from build123d import *

# Parameters (mm, degrees)
F1_DEPTH = 20.6
F2_R     = 5


with BuildPart() as f1:
    # F0 (on Front) → F1 (new body, symmetric)
    with BuildSketch(Plane.XZ):
        Polygon((-82.7489259505, 37), (-107.7489259505, 37), (-107.7489259505, -54.4), (-83.9489259505, -54.4), (-67.4489259505, -25), (-7.4489259505, -25), (-7.4489259505, 67), (-34.7489259505, 67), (-34.7489259505, 0), (-82.7489259505, 0), align=None)
    extrude(amount=F1_DEPTH, both=True)

    # F2
    f2_edges = [f1.edges().sort_by_distance(p)[0] for p in [
        (-107.748926, 0, 37),
        (-82.748926, 0, 37),
        (-95.248926, -20.6, 37),
        (-95.248926, 20.6, 37),
        (-82.748926, -20.6, 18.5),
        (-82.748926, 0, 0),
        (-82.748926, 20.6, 18.5),
        (-58.748926, 20.6, 0),
        (-58.748926, -20.6, 0),
        (-34.748926, 0, 0),
        (-34.748926, 0, 67),
        (-21.098926, -20.6, 67),
        (-21.098926, 20.6, 67),
        (-7.448926, 0, 67),
        (-34.748926, -20.6, 33.5),
        (-7.448926, -20.6, 21),
        (-7.448926, 20.6, 21),
        (-107.748926, -20.6, -8.7),
        (-107.748926, 20.6, -8.7),
        (-34.748926, 20.6, 33.5),
    ]]
    fillet(f2_edges, radius=F2_R)


solid = f1.part
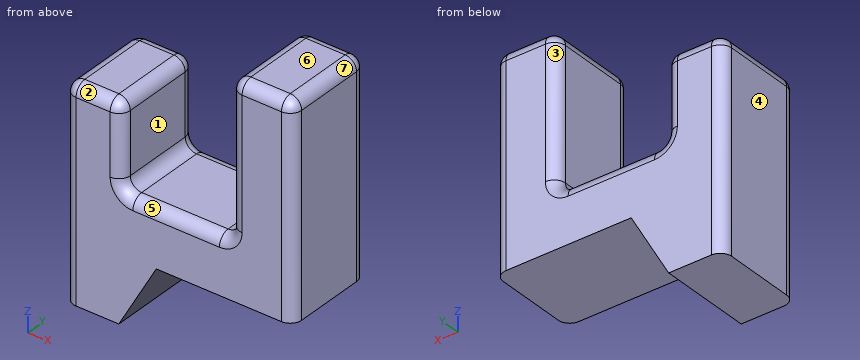
Can you work these out from the model? Positions are in its coordinate system, mm. Face numbers are marked on the shaded views. A direction names the side the tool comes from. Give positions to 0.01 mm unless a question says otherwise; leave off trailing zeros. Order: outer loops, then holes, each group sorted by start corner. A loop starts at its lowest first (then second) coordinate and runs counter-clockwise, first axis right, second up. Notation, with made-up numbers: M 5.5,46.25 L 23.5,46.25 A6 ccw 23.5,57.25 Z; hole C -26,-30.5 d1. An arc over 180 degrees is marked long. Use one line per item in the form item = value. Start each with the question number.
Item 1: If we section it at D-D (x = -45): Write out the boundary of the cut face in (y, z).
Item 2: If I drill on line 1 along X through (y, z) = (11, 9.5); line 2 along X through (y, z) = (16, 8); line 3 along X through (y, z) = (5, 40), over which ranges is the centre line in solid material (lowest first)?
Item 3: If we section it at B-B (z = 52.5): Write out the boundary of the cut face in (x, y).
Item 4: We'd pull the mould along X, two halves only. Please class the marked faces 4, 5, 6 and 7: +X half, -X half, draft (parallel to the pull), parting line (faces both ways), or undercut.
Item 5: If we section it at A-A (z = 7): Write out the boundary of the cut face in (x, y), then the cut area to 3 significant figures.
Item 6: If we section it at C-C (y = -1.5): Write out the boundary of the cut face in (x, z).
Item 7: Will these pins go through, and if not, where does the flat tip stop? pin 1 Ø15.5 at (x, y) = (-56, 8) entering from +Z; pin 2 Ø3 at (x, z) = (-84, 28) entering from -Y; pin 3 Ø4.5 at (x, y) = (-98, -7) entering from +Z.
Item 8: For the marked faces 1, 2 and 3, which set-ups out of +Z, -Z, +X, -X, +Y, -Y let a thin tool reach every point of the face, with its end or its side?
Outcome:
q1.outline = M -20.6,-25 L 20.6,-25 L 20.6,-5 A5 ccw 15.6,0 L -15.6,0 A5 ccw -20.6,-5 Z
q2.line_1 = -107.75 to -82.75, -34.75 to -7.45
q2.line_2 = -107.73 to -82.76, -34.73 to -7.46
q2.line_3 = -34.75 to -7.45
q3.outline = M -34.75,-15.6 A5 ccw -29.75,-20.6 L -12.45,-20.6 A5 ccw -7.45,-15.6 L -7.45,15.6 A5 ccw -12.45,20.6 L -29.75,20.6 A5 ccw -34.75,15.6 Z
q4.face_4 = -X half
q4.face_5 = undercut
q4.face_6 = draft
q4.face_7 = +X half
q5.outline = M -107.75,-15.6 A5 ccw -102.75,-20.6 L -87.75,-20.6 A5 ccw -82.75,-15.6 L -82.75,15.6 A5 ccw -87.75,20.6 L -102.75,20.6 A5 ccw -107.75,15.6 Z; M -34.75,-15.6 A5 ccw -29.75,-20.6 L -12.45,-20.6 A5 ccw -7.45,-15.6 L -7.45,15.6 A5 ccw -12.45,20.6 L -29.75,20.6 A5 ccw -34.75,15.6 Z
q5.area = 2,110 mm2
q6.outline = M -107.75,-54.4 L -83.95,-54.4 L -67.45,-25 L -7.45,-25 L -7.45,62 A5 ccw -12.45,67 L -29.75,67 A5 ccw -34.75,62 L -34.75,5 A5 cw -39.75,0 L -77.75,0 A5 cw -82.75,5 L -82.75,32 A5 ccw -87.75,37 L -102.75,37 A5 ccw -107.75,32 Z
q7.pin_1 = 0
q7.pin_2 = -20.07
q7.pin_3 = 37
q8.face_1 = +Z, +Y, -Y
q8.face_2 = +Z, -X, -Y
q8.face_3 = +Z, +Y
